Source: CAD feature listing. Evaluate the final solid. Frame: model axes, mm. A direction names the side the tool comes from. Round coordinates to 2 decimals unless told otherwise and drop trailing zeros. Write each loop counter-clockwise with the first axis right and the second up, starting at its lowest first coordinate (ties: lowest second). Pieces come first, ordered by that corner, then holes.
Autodesk Inventor part; units mm, degrees
ref_plane "YZ Plane" through (0, 0, 0) normal (1, 0, 0) x (0, 1, 0)
ref_plane "XZ Plane" through (0, 0, 0) normal (0, 1, 0) x (-1, 0, 0)
ref_plane "XY Plane" through (0, 0, 0) normal (0, 0, 1) x (1, 0, 0)
sketch "スケッチ1" plane through (0, 0, 0) normal (0, 0, 1) x (1, 0, 0)
  line L0 (-45, 45) -> (45, 45)
  line L1 (45, 45) -> (45, -45)
  line L2 (45, -45) -> (-45, -45)
  line L3 (-45, -45) -> (-45, 45)
  point P0 (0, 0)
  point P1 (0, 45)
  point P2 (-45, 0)
  dimension "d0" = 90
  dimension "d1" = 90
extrude "押し出し1" add sketch "スケッチ1" along normal blind 180
sketch "スケッチ2" plane through (0, 0, 180) normal (0, 0, 1) x (1, 0, 0)
  point P0 (0, 0)
sketch "スケッチ3" plane through (0, 0, 180) normal (0, 0, 1) x (1, 0, 0)
  circle A0 centre (0, 0) radius 42
  dimension "d4" = 84
extrude "押し出し2" cut sketch "スケッチ3" against normal through all keep common part
sketch "スケッチ4" plane through (0, 0, 180) normal (0, 0, 1) x (1, 0, 0)
  circle A0 centre (0, 0) radius 34
  circle A1 centre (0, 0) radius 42 construction
  dimension "d7" = 8
extrude "押し出し3" cut sketch "スケッチ4" against normal blind 100
sketch "スケッチ5" plane through (0, 0, 0) normal (0, 0, -1) x (-1, 0, 0)
  circle A0 centre (0, 0) radius 42
extrude "押し出し4" cut sketch "スケッチ5" against normal blind 60
fillet "フィレット1" radius 20 1 edges at (-34, 0, 80)
sketch "スケッチ6" plane through (0, 0, 60) normal (0, 0, -1) x (-1, 0, 0)
  circle A0 centre (0, 0) radius 34
extrude "押し出し5" cut sketch "スケッチ6" against normal blind 8
fillet "フィレット2" radius 4 4 edges at (-42, 0, 180) (-34, 0, 180) (-42, 0, 60) (34, 0, 60)
fillet "フィレット3" radius 20 1 edges at (34, 0, 68)
equation "\"d1\" = d0"
properties part number "cup" material "アルミニウム 6061"
1) Material intervals for line 1 (Y direction, x = 0, z = 130); line 2 (Y direction, x = 3.5, z = 96); line 3 (Z direction, x = 2, y = 4.5), sorted ascending.
Taken from the geometry:
line 1: y = -42 to -34, 34 to 42
line 2: y = -41.85 to -33.41, 33.41 to 41.85
line 3: z = 68 to 80
2) Reachability of faces 3 (the face through (0, 0, 80)), 4 (the face through (0, 0, 68)) from +Z, -Z, +X, -X, +Y, -Y: full face, straight path, thin tool, end or side. Return the list, or none.
Taken from the geometry:
face 3: +Z
face 4: -Z
3) Pull-direction query (X, two-part tool) for faces 1 (the face through (40.06, 12.62, 120.78)), 2 (the face through (18.28, 28.67, 138.53)); classes: released by +X, released by -X, zero draft, split by the parting line, or undercut.
Taken from the geometry:
face 1: split by the parting line
face 2: undercut
4) Section query B-B on z = 75. Return the cut outline in (x, y), then the cut area to 3 significant figures.
Taken from the geometry:
outline: circle Ø84 at (0, 0)
area: 5,540 mm2
5) Contact query for flat-ended pins moving along their axis: P1, Ø2, axis at x = 5, y = -13, coming from the -Z side; P2, Ø1.5, axis at x = -27.5, z = 164, coming from the -Y side; P3, Ø1.5, axis at y = -19.5, z = 156.5, coming from the -X side. Output: stop coordinate, or through.
Taken from the geometry:
P1: stops at z = 68
P2: stops at y = -32.38
P3: stops at x = -37.58
6) Section query A-A on z = 161. Return the cut outline in (x, y).
Taken from the geometry:
outline: circle Ø84 at (0, 0); hole circle Ø68 at (0, 0)
